```python
from build123d import *

# Parameters (mm, degrees)
ESQUISSE1_R             = 4.55
ESQUISSE1_R_2           = 2.9
BOSS_EXTRU_1_DEPTH      = 12
BOSS_EXTRU_2_START      = -19.2
ESQUISSE1_3_R           = 4.9
ESQUISSE1_3_R_2         = 4.55
ESQUISSE1_3_R_3         = 2.9
BOSS_EXTRU_2_DEPTH      = 19.2
ESQUISSE2_W             = 6.768135737
ESQUISSE2_H             = 1.1
ENL_V_MAT_EXTRU_1_DEPTH = 5
R_VOLUTION1_ANGLE       = 180


with BuildPart() as part:
    # Esquisse1 → Boss.-Extru.1 (new body)
    with BuildSketch(Plane.XY):
        Circle(ESQUISSE1_R)
        Circle(ESQUISSE1_R_2, mode=Mode.SUBTRACT)
    extrude(amount=BOSS_EXTRU_1_DEPTH)

    # Esquisse1_3 → Boss.-Extru.2 (add)
    # profile 1 of 2: a face of its own
    with BuildSketch(Plane.XY.offset(BOSS_EXTRU_2_START)):
        Circle(ESQUISSE1_3_R)
        Circle(ESQUISSE1_3_R_2, mode=Mode.SUBTRACT)
    # profile 2 of 2: a face of its own
    with BuildSketch(Plane.XY.offset(BOSS_EXTRU_2_START)):
        Circle(ESQUISSE1_3_R_2)
        Circle(ESQUISSE1_3_R_3, mode=Mode.SUBTRACT)
    extrude(amount=BOSS_EXTRU_2_DEPTH)

    # Esquisse2 → Enl_v. mat.-Extru.1 (cut, symmetric)
    with BuildSketch(Plane(origin=(0, 0, 0), x_dir=(1, 0, 0), z_dir=(0, 1, 0))):
        with Locations((3.384067869, 18.65)):
            Rectangle(ESQUISSE2_W, ESQUISSE2_H)
    extrude(amount=ENL_V_MAT_EXTRU_1_DEPTH, both=True, mode=Mode.SUBTRACT)

    # Esquisse3 → R_volution1 (revolve)
    with BuildSketch(Plane(origin=(0, 0, 0), x_dir=(0, 0, -1), z_dir=(1, 0, 0))):
        Polygon((18.9, -4.9), (19.2, -4.9), (19.2, -4), (20.1, -4), (20.1, -5.3), (18.9, -5.3), align=None)
    revolve(axis=Axis((0, 0, 0), (0, 0, -1)), revolution_arc=R_VOLUTION1_ANGLE)


solid = part.part
```
Build history of the part. All positions in model axes, mm. A direction names the side the tool comes from. Coordinates: 2 decimals unless noted, no trailing zeros. Write each loop counter-clockwise with the first axis right and the second up, starting at its lowest first coordinate (ties: lowest second). Pieces come first, ordered by that corner, then holes.
1. 3-axis set-ups, long thin cutter, end or side, ignore diameter. For faces 1 (the flat face through (-5, -1, -18.9)), 2 (the flat face through (0, 4, -19)), 3 (the cylindrical face through (-0.99, -4.44, 5.92)): which of +Z, -Z, +X, -X, +Y, -Y reach the whole face in a straight line?
Answer block:
face 1: +Z, -X
face 2: -Z, +X, +Y, -Y
face 3: +Z
2. Band-saw the part on B-B, the plane z = -0.5. Give the cut face in (x, y), and give its area (3 significant figures).
Answer block:
outline: circle Ø9.8 at (0, 0); hole circle Ø5.8 at (0, 0)
area: 49.0 mm2
3. Drop flat-ended pins along their axis: pin 1 (1.6 mm diameter, centred on y = -4, z = -19, fed in from +X); pin 2 (1 mm diameter, centred on y = 3, z = 4, fed in from -X); pin 3 (6 mm diameter, centred on y = -3.5, z = -1.5, fed in from -X). Give the stop position or say it passes through.
Answer block:
pin 1: stops at x = 0
pin 2: stops at x = -3.8
pin 3: stops at x = -4.87
4. Band-saw the part on C-C, the plane x = 2.25. Give the cut face in (y, z), and give its area (3 significant figures).
Answer block:
outline: (-4.35, -18.1) - (-1.83, -18.1) - (-1.83, 12) - (-3.95, 12) - (-3.95, 0) - (-4.35, 0) - close; (1.83, -18.1) - (4.35, -18.1) - (4.35, 0) - (3.95, 0) - (3.95, 12) - (1.83, 12) - close
area: 142 mm2
5. Pull direction Y, two halves, no side cores. Call faces 4 (the cylindrical face through (-4, -0.1, -19.7)), 5 (the flat face through (-3, 1, -19.2)), 6 (the cylindrical face through (-5.3, -0.1, -19.5)), 7 (the flat face through (0, -4, -19)): released by +Y, released by -Y, zero draft, split by the parting line, or undercut.
Answer block:
face 4: undercut
face 5: undercut
face 6: split by the parting line
face 7: zero draft
6. Drill centre lines: probe 1 along Y at (x, z) = (0, -2); probe 2 along Y at (x, z) = (0, 9.5). Where is each one in solid material? Low to high.
Answer block:
probe 1: y = -4.9 to -2.9, 2.9 to 4.9
probe 2: y = -4.55 to -2.9, 2.9 to 4.55
7. Band-saw the part on A-A, the plane y = 1. Give the cut face in (x, z).
Answer block:
outline: (-5.2, -20.1) - (-3.87, -20.1) - (-3.87, -19.2) - (-2.72, -19.2) - (-2.72, 12) - (-4.44, 12) - (-4.44, 0) - (-4.8, 0) - (-4.8, -18.9) - (-5.2, -18.9) - close; (2.72, -18.1) - (4.8, -18.1) - (4.8, 0) - (4.44, 0) - (4.44, 12) - (2.72, 12) - close
8. Band-saw the part on D-D, the plane x = 3.5. Give the cut face in (y, z).
Answer block:
outline: (-3.43, -18.1) - (3.43, -18.1) - (3.43, 0) - (2.91, 0) - (2.91, 12) - (-2.91, 12) - (-2.91, 0) - (-3.43, 0) - close
